For this review, take the finished solid that the model builds, in its own axes (mm). Face numbers are marked on the shaded views. A direction names the side the tool comes from. Give positions to 0.01 mm unless a question says otherwise; leave off trailing zeros. Write each loop counter-clockwise with the first axis right and the second up, starting at its lowest first coordinate (ties: lowest second). Pieces come first, ordered by that corner, then holes.
1) Wall thickness on line 1 along X through (y, z) = (5, -23); line 2 along Z through (x, y) = (0, 15.65): over which ranges is each line inside the solid? List them lowest first.
2) We need section C-C on x = 0. Give the boundary of the cut face in (y, z).
3) Machinability: for the marked faces 1 and 2, which of the approach directions +Z, -Z, +X, -X, +Y, -Y give a long, thin tool a straight path to every point of the face, cutting with its end or side? Answer none if there is none.
4) Draft analysis for pull direction Y (two halves, no side actions). For the marked faces 3, 4 and 5, state which applies: pulls with the +Y half, pulls with the -Y half, needs draft (parallel to the pull), parting line crosses it, or undercut.
5) We need section A-A on x = -8.5. Give the boundary of the cut face in (y, z), and give its area (3 significant figures).
6) For P1, Ø6, axis at x = -11, y = 0, coming from the +Z side; P2, Ø20.5, axis at x = 0, z = -12.7, coming from the +Y side, all flat-tipped, find the tip position at first contact; note any pin that passes through.
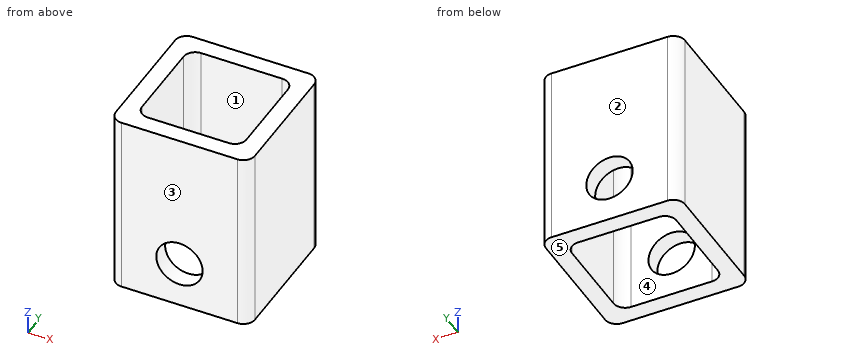
from build123d import *

# Parameters (mm, degrees)
F0_W     = 38.1
F0_H     = 38.1
F0_W_2   = 28.575
F0_H_2   = 28.575
F1_DEPTH = 25.4
F2_R     = 3.175
F3_R     = 6.35
F4_DEPTH = 38.1


with BuildPart() as f1:
    # F0 (on Top) → F1 (new body, symmetric)
    with BuildSketch(Plane.XY):
        Rectangle(F0_W, F0_H)
        Rectangle(F0_W_2, F0_H_2, mode=Mode.SUBTRACT)
    extrude(amount=F1_DEPTH, both=True)

    # F2
    f2_edges = [f1.edges().sort_by_distance(p)[0] for p in [
        (19.05, -19.05, 0),
        (-19.05, -19.05, 0),
        (-14.2875, 14.2875, 0),
        (14.2875, 14.2875, 0),
        (-19.05, 19.05, 0),
        (19.05, 19.05, 0),
        (-14.2875, -14.2875, 0),
        (14.2875, -14.2875, 0),
    ]]
    fillet(f2_edges, radius=F2_R)

    # F3 (on face) → F4 (cut, through all)
    with BuildSketch(Plane.XZ.offset(19.05)):
        with Locations((0, -12.7)):
            Circle(F3_R)
    extrude(amount=-F4_DEPTH, mode=Mode.SUBTRACT)


solid = f1.part
Results list:
1. line 1: x = -19.05 to -14.29, 14.29 to 19.05
1. line 2: z = -25.4 to -19.05, -6.35 to 25.4
2. outline: (-19.05, -25.4) - (-14.29, -25.4) - (-14.29, -19.05) - (-19.05, -19.05) - close; (-19.05, -6.35) - (-14.29, -6.35) - (-14.29, 25.4) - (-19.05, 25.4) - close; (14.29, -25.4) - (19.05, -25.4) - (19.05, -19.05) - (14.29, -19.05) - close; (14.29, -6.35) - (19.05, -6.35) - (19.05, 25.4) - (14.29, 25.4) - close
3. face 1: +Z, -Z
3. face 2: +Z, -Z, +X, -X, +Y
4. face 3: pulls with the -Y half
4. face 4: undercut
4. face 5: needs draft
5. outline: (-19.05, -25.4) - (-14.29, -25.4) - (-14.29, 25.4) - (-19.05, 25.4) - close; (14.29, -25.4) - (19.05, -25.4) - (19.05, 25.4) - (14.29, 25.4) - close
5. area: 484 mm2
6. P1: passes through
6. P2: stops at y = 19.05
